Build history of the part. All positions in model axes, mm. Round coordinates to 2 decimals unless told otherwise and drop trailing zeros. Write each loop counter-clockwise with the first axis right and the second up, starting at its lowest first coordinate (ties: lowest second). Pieces come first, ordered by that corner, then holes. Notation, with made-up numbers: (-13.75, 75) - (10.25, 75) arc R34 cw to (10.25, 109) - close; hole circle Ø6 at (35.5, -13.75). An arc over 180 degrees is marked (long way). One line per question, with ' | ' between items.
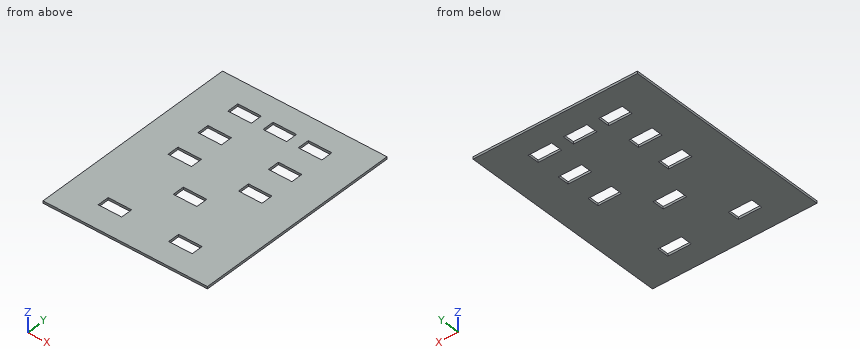
from build123d import *

# Parameters (mm, degrees)
SKETCH1_W           = 350
SKETCH1_H           = 450
BOSS_EXTRUDE1_DEPTH = 5
SKETCH2_W           = 50
SKETCH2_H           = 25
CUT_EXTRUDE1_DEPTH  = 571.109638578


with BuildPart() as part:
    # Sketch1 → Boss-Extrude1 (new body)
    with BuildSketch(Plane.XY):
        with Locations((175, 225)):
            Rectangle(SKETCH1_W, SKETCH1_H)
    extrude(amount=BOSS_EXTRUDE1_DEPTH)

    # Sketch2 → Cut-Extrude1 (cut, through all)
    with BuildSketch(Plane.XY.offset(5)):
        with Locations((100, 387.5)):
            Rectangle(SKETCH2_W, SKETCH2_H)
    cut_extrude1 = extrude(amount=-CUT_EXTRUDE1_DEPTH, mode=Mode.SUBTRACT)

    # Sketch-Pattern1: Cut-Extrude1 at 9 more places
    with Locations((75, 0, 0), (150, 0, 0), (0, -75, 0), (0, -150, 0), (0, -325, 0), (150, -75, 0), (150, -150, 0), (75, -225, 0), (150, -325, 0)):
        add(cut_extrude1, mode=Mode.SUBTRACT)


solid = part.part
Q1. Saw through at D-D, the plane z = 1.3. State how many separate pieces and enclosed holes the cut face has, then the cut area to 3 significant figures.
Found:
separate pieces: 1 | enclosed holes: 10 | area: 145,000 mm^2
Q2. Saw through at C-C, the plane y = 385. List the corners of the cut face in (x, z), then the cut area to 3 significant figures.
Found:
outline: (0, 0) - (75, 0) - (75, 5) - (0, 5) - close; (125, 0) - (150, 0) - (150, 5) - (125, 5) - close; (200, 0) - (225, 0) - (225, 5) - (200, 5) - close; (275, 0) - (350, 0) - (350, 5) - (275, 5) - close | area: 1,000 mm^2
Q3. Saw through at A-A, the plane x = 184. List the corners of the cut face in (y, z), then the cut area to 3 significant figures.
Found:
outline: (0, 0) - (150, 0) - (150, 5) - (0, 5) - close; (175, 0) - (375, 0) - (375, 5) - (175, 5) - close; (400, 0) - (450, 0) - (450, 5) - (400, 5) - close | area: 2,000 mm^2
Q4. Saw through at B-B, the plane x = 112.5. List the corners of the cut face in (y, z).
Found:
outline: (0, 0) - (50, 0) - (50, 5) - (0, 5) - close; (75, 0) - (225, 0) - (225, 5) - (75, 5) - close; (250, 0) - (300, 0) - (300, 5) - (250, 5) - close; (325, 0) - (375, 0) - (375, 5) - (325, 5) - close; (400, 0) - (450, 0) - (450, 5) - (400, 5) - close
Q5. Drill centre lines: L1, parallel to Y at x = 85.5, z = 2.2; L2, parallel to X at y = 64, z = 2.9; L3, parallel to X at y = 392, z = 0.85. Where is each one in solid material? Low to high. Write a range as from..to.
Found:
L1: 0..50, 75..225, 250..300, 325..375, 400..450 | L2: 0..75, 125..225, 275..350 | L3: 0..75, 125..150, 200..225, 275..350
